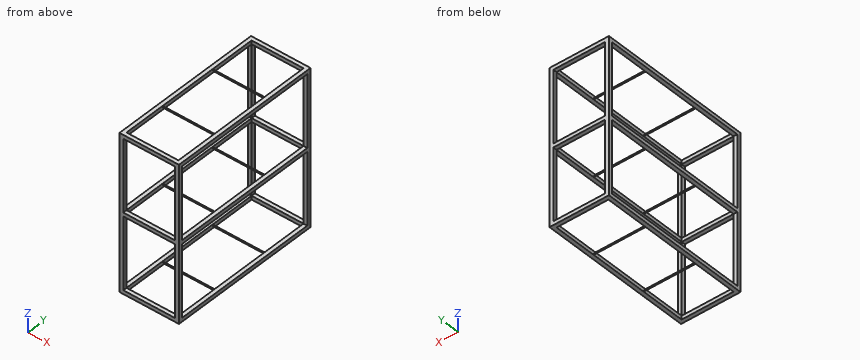
from build123d import *

# Parameters (mm, degrees)
SKETCH1_W             = 40
SKETCH1_H             = 40
SKETCH1_W_2           = 36
SKETCH1_H_2           = 36
BOSS_EXTRUDE1_DEPTH   = 825
BOSS_EXTRUDE1_2_DEPTH = 825
SKETCH2_W             = 40
SKETCH2_H             = 40
SKETCH2_W_2           = 36
SKETCH2_H_2           = 36
BOSS_EXTRUDE2_DEPTH   = 550
SKETCH3_W             = 40
SKETCH3_H             = 40
SKETCH3_W_2           = 36
SKETCH3_H_2           = 36
BOSS_EXTRUDE5_DEPTH   = 1551.5
SKETCH5_W             = 40
SKETCH5_H             = 40
SKETCH5_W_2           = 38
SKETCH5_H_2           = 38
BOSS_EXTRUDE6_DEPTH   = 1650
SKETCH6_W             = 40
SKETCH6_H             = 40
SKETCH6_W_2           = 38
SKETCH6_H_2           = 38
BOSS_EXTRUDE7_DEPTH   = 550
SKETCH7_R             = 6
BOSS_EXTRUDE8_DEPTH   = 550
SKETCH8_W             = 40
SKETCH8_H             = 40
BOSS_EXTRUDE10_DEPTH  = 1
SKETCH9_W             = 40
SKETCH9_H             = 40
BOSS_EXTRUDE11_DEPTH  = 1


with BuildPart() as part:
    # Sketch1 → Boss-Extrude1 (new, symmetric)
    with BuildSketch(Plane.XY):
        with Locations((-295, 20)):
            Rectangle(SKETCH1_W, SKETCH1_H)
        with Locations((-295, 20)):
            Rectangle(SKETCH1_W_2, SKETCH1_H_2, mode=Mode.SUBTRACT)
    extrude(amount=BOSS_EXTRUDE1_DEPTH, both=True)



with BuildPart() as body_2:
    # Sketch1 → Boss-Extrude1 2 (new, symmetric)
    with BuildSketch(Plane.XY):
        with Locations((295, 20)):
            Rectangle(SKETCH1_W, SKETCH1_H)
        with Locations((295, 20)):
            Rectangle(SKETCH1_W_2, SKETCH1_H_2, mode=Mode.SUBTRACT)
    extrude(amount=BOSS_EXTRUDE1_2_DEPTH, both=True)


with BuildPart() as part_1:
    add(part.part)

    add(body_2.part)  # Boss-Extrude2 merges body 2
    # Sketch2 → Boss-Extrude2 (add)
    # profile 1 of 3: a face of its own
    with BuildSketch(Plane(origin=(-275, 0, 0), x_dir=(0, 0, -1), z_dir=(1, 0, 0))):
        with Locations((-805, 20)):
            Rectangle(SKETCH2_W, SKETCH2_H)
        with Locations((-805, 20)):
            Rectangle(SKETCH2_W_2, SKETCH2_H_2, mode=Mode.SUBTRACT)
    # profile 2 of 3: a face of its own
    with BuildSketch(Plane(origin=(-275, 0, 0), x_dir=(0, 0, -1), z_dir=(1, 0, 0))):
        with Locations((805, 20)):
            Rectangle(SKETCH2_W, SKETCH2_H)
        with Locations((805, 20)):
            Rectangle(SKETCH2_W_2, SKETCH2_H_2, mode=Mode.SUBTRACT)
    # profile 3 of 3: a face of its own
    with BuildSketch(Plane(origin=(-275, 0, 0), x_dir=(0, 0, -1), z_dir=(1, 0, 0))):
        with Locations((0, 20)):
            Rectangle(SKETCH2_W, SKETCH2_H)
        with Locations((0, 20)):
            Rectangle(SKETCH2_W_2, SKETCH2_H_2, mode=Mode.SUBTRACT)
    extrude(amount=BOSS_EXTRUDE2_DEPTH)

    # Sketch3 → Boss-Extrude5 (add)
    # profile 1 of 6: a face of its own
    with BuildSketch(Plane(origin=(0, 40, 0), x_dir=(1, 0, 0), z_dir=(0, 1, 0))):
        with Locations((-295, -805)):
            Rectangle(SKETCH3_W, SKETCH3_H)
        with Locations((-295, -805)):
            Rectangle(SKETCH3_W_2, SKETCH3_H_2, mode=Mode.SUBTRACT)
    # profile 2 of 6: a face of its own
    with BuildSketch(Plane(origin=(0, 40, 0), x_dir=(1, 0, 0), z_dir=(0, 1, 0))):
        with Locations((295, -805)):
            Rectangle(SKETCH3_W, SKETCH3_H)
        with Locations((295, -805)):
            Rectangle(SKETCH3_W_2, SKETCH3_H_2, mode=Mode.SUBTRACT)
    # profile 3 of 6: a face of its own
    with BuildSketch(Plane(origin=(0, 40, 0), x_dir=(1, 0, 0), z_dir=(0, 1, 0))):
        with Locations((295, 0)):
            Rectangle(SKETCH3_W, SKETCH3_H)
        with Locations((295, 0)):
            Rectangle(SKETCH3_W_2, SKETCH3_H_2, mode=Mode.SUBTRACT)
    # profile 4 of 6: a face of its own
    with BuildSketch(Plane(origin=(0, 40, 0), x_dir=(1, 0, 0), z_dir=(0, 1, 0))):
        with Locations((-295, 0)):
            Rectangle(SKETCH3_W, SKETCH3_H)
        with Locations((-295, 0)):
            Rectangle(SKETCH3_W_2, SKETCH3_H_2, mode=Mode.SUBTRACT)
    # profile 5 of 6: a face of its own
    with BuildSketch(Plane(origin=(0, 40, 0), x_dir=(1, 0, 0), z_dir=(0, 1, 0))):
        with Locations((-295, 805)):
            Rectangle(SKETCH3_W, SKETCH3_H)
        with Locations((-295, 805)):
            Rectangle(SKETCH3_W_2, SKETCH3_H_2, mode=Mode.SUBTRACT)
    # profile 6 of 6: a face of its own
    with BuildSketch(Plane(origin=(0, 40, 0), x_dir=(1, 0, 0), z_dir=(0, 1, 0))):
        with Locations((295, 805)):
            Rectangle(SKETCH3_W, SKETCH3_H)
        with Locations((295, 805)):
            Rectangle(SKETCH3_W_2, SKETCH3_H_2, mode=Mode.SUBTRACT)
    extrude(amount=BOSS_EXTRUDE5_DEPTH)

    # Sketch5 → Boss-Extrude6 (add)
    # profile 1 of 2: a face of its own
    with BuildSketch(Plane.XY.offset(825)):
        with Locations((-295, 1611.5)):
            Rectangle(SKETCH5_W, SKETCH5_H)
        with Locations((-295, 1611.5)):
            Rectangle(SKETCH5_W_2, SKETCH5_H_2, mode=Mode.SUBTRACT)
    # profile 2 of 2: a face of its own
    with BuildSketch(Plane.XY.offset(825)):
        with Locations((295, 1611.5)):
            Rectangle(SKETCH5_W, SKETCH5_H)
        with Locations((295, 1611.5)):
            Rectangle(SKETCH5_W_2, SKETCH5_H_2, mode=Mode.SUBTRACT)
    extrude(amount=-BOSS_EXTRUDE6_DEPTH)

    # Sketch6 → Boss-Extrude7 (add)
    # profile 1 of 3: a face of its own
    with BuildSketch(Plane(origin=(-275, 0, 0), x_dir=(0, 0, -1), z_dir=(1, 0, 0))):
        with Locations((0, 1611.5)):
            Rectangle(SKETCH6_W, SKETCH6_H)
        with Locations((0, 1611.5)):
            Rectangle(SKETCH6_W_2, SKETCH6_H_2, mode=Mode.SUBTRACT)
    # profile 2 of 3: a face of its own
    with BuildSketch(Plane(origin=(-275, 0, 0), x_dir=(0, 0, -1), z_dir=(1, 0, 0))):
        with Locations((-805, 1611.5)):
            Rectangle(SKETCH6_W, SKETCH6_H)
        with Locations((-805, 1611.5)):
            Rectangle(SKETCH6_W_2, SKETCH6_H_2, mode=Mode.SUBTRACT)
    # profile 3 of 3: a face of its own
    with BuildSketch(Plane(origin=(-275, 0, 0), x_dir=(0, 0, -1), z_dir=(1, 0, 0))):
        with Locations((805, 1611.5)):
            Rectangle(SKETCH6_W, SKETCH6_H)
        with Locations((805, 1611.5)):
            Rectangle(SKETCH6_W_2, SKETCH6_H_2, mode=Mode.SUBTRACT)
    extrude(amount=BOSS_EXTRUDE7_DEPTH)

    # Sketch7 → Boss-Extrude8 (add)
    with BuildSketch(Plane.ZY.offset(-275)):
        with Locations(Location((805, 1119, 0), (0, 0, 180))):
            Circle(SKETCH7_R)
        with Locations(Location((805, 499, 0), (0, 0, 180))):
            Circle(SKETCH7_R)
        with Locations(Location((0, 1119, 0), (0, 0, 180))):
            Circle(SKETCH7_R)
        with Locations(Location((0, 499, 0), (0, 0, 180))):
            Circle(SKETCH7_R)
        with Locations(Location((-805, 499, 0), (0, 0, 180))):
            Circle(SKETCH7_R)
        with Locations(Location((-805, 1119, 0), (0, 0, 180))):
            Circle(SKETCH7_R)
    extrude(amount=BOSS_EXTRUDE8_DEPTH)

    # Sketch8 → Boss-Extrude10 (add)
    with BuildSketch(Plane.XY.offset(825)):
        with Locations((-295, 1611.5)):
            Rectangle(SKETCH8_W, SKETCH8_H)
        with Locations((295, 1611.5)):
            Rectangle(SKETCH8_W, SKETCH8_H)
        with Locations((-295, 20)):
            Rectangle(SKETCH8_W, SKETCH8_H)
        with Locations((295, 20)):
            Rectangle(SKETCH8_W, SKETCH8_H)
    extrude(amount=-BOSS_EXTRUDE10_DEPTH)

    # Sketch9 → Boss-Extrude11 (add)
    with BuildSketch(Plane(origin=(0, 0, -825), x_dir=(-1, 0, 0), z_dir=(0, 0, -1))):
        with Locations((-295, 1611.5)):
            Rectangle(SKETCH9_W, SKETCH9_H)
        with Locations((295, 1611.5)):
            Rectangle(SKETCH9_W, SKETCH9_H)
        with Locations((295, 20)):
            Rectangle(SKETCH9_W, SKETCH9_H)
        with Locations((-295, 20)):
            Rectangle(SKETCH9_W, SKETCH9_H)
    extrude(amount=-BOSS_EXTRUDE11_DEPTH)


solid = part_1.part
Model file for the job. Use its own axes, mm. Coordinates: 2 decimals unless noted, no trailing zeros. One line per item, written item: value. Start each with the question number.
1) Flat gauge pin, fed straight in: pin 1 Ø3 at (x, y) = (233.5, 507) entering from +Z. Where does the tip first touch, or does it go through?
2) Probe probe 1 along Y at (x, z) = (281, -31); probe 2 along X at (y, z) = (1038, -12). List the from-to ranges inside material, lowest first.
3) Slice it at A-A on z = 612. Count the separate pieces of the cut face and the enclosed holes in it, then the cut area to 3 significant figures.
Answers follow:
1. pin 1: through
2. probe 1: 0 to 2, 38 to 40, 1591.5 to 1592.5, 1630.5 to 1631.5
2. probe 2: -315 to -313, -277 to -275, 275 to 277, 313 to 315
3. separate pieces: 4
3. enclosed holes: 4
3. area: 920 mm2
